```python
from build123d import *

# Parameters (mm, degrees)
SKETCH_1_W          = 20
SKETCH_1_H          = 145
EXTRUDE_1_DEPTH     = 5
SKETCH_3_W          = 20
SKETCH_3_H          = 5
EXTRUDE_2_DEPTH     = 50
SKETCH_4_W          = 20
SKETCH_4_H          = 5
EXTRUDE_3_DEPTH     = 30
SKETCH_5_W          = 20
SKETCH_5_H          = 20
CUT_EXTRUDE_1_DEPTH = 30
SKETCH_6_W          = 20
SKETCH_6_H          = 5
EXTRUDE_4_DEPTH     = 20
SKETCH_7_W          = 20
SKETCH_7_H          = 5
EXTRUDE_5_DEPTH     = 20
EXTRUDE_6_DEPTH     = 2.5
SKETCH_10_R         = 2
CUT_EXTRUDE_2_DEPTH = 5
SKETCH_11_R         = 2
CUT_EXTRUDE_3_DEPTH = 5
SKETCH_12_R         = 2.75
CUT_EXTRUDE_4_DEPTH = 5
SKETCH_13_W         = 20
SKETCH_13_H         = 5
EXTRUDE_7_DEPTH     = 5
SKETCH_14_W         = 20
SKETCH_14_H         = 5
EXTRUDE_8_DEPTH     = 20
SKETCH_15_R         = 2.75
CUT_EXTRUDE_5_DEPTH = 20
SKETCH_16_W         = 20
SKETCH_16_H         = 5
EXTRUDE_9_DEPTH     = 75.52
SKETCH_17_W         = 5
SKETCH_17_H         = 20
EXTRUDE_10_DEPTH    = 20
SKETCH_18_R         = 2.6
CUT_EXTRUDE_6_DEPTH = 20


with BuildPart() as part:
    # 草图1 → 凸台-拉伸1 (new body)
    with BuildSketch(Plane.XY):
        with Locations((0.170940171, -57.628205128)):
            Rectangle(SKETCH_1_W, SKETCH_1_H)
    extrude(amount=-EXTRUDE_1_DEPTH)

    # 草图3 → 凸台-拉伸2 (add)
    with BuildSketch(Plane(origin=(0, 0, -5), x_dir=(-1, 0, 0), z_dir=(0, 0, -1))):
        with Locations((-0.170940171, 12.371794872)):
            Rectangle(SKETCH_3_W, SKETCH_3_H)
    extrude(amount=EXTRUDE_2_DEPTH)

    # 草图4 → 凸台-拉伸3 (add)
    with BuildSketch(Plane(origin=(0, 0, -5), x_dir=(-1, 0, 0), z_dir=(0, 0, -1))):
        with Locations((-0.170940171, -107.628205128)):
            Rectangle(SKETCH_4_W, SKETCH_4_H)
    extrude(amount=EXTRUDE_3_DEPTH)

    # 草图5 → 切除-拉伸1 (cut)
    with BuildSketch(Plane(origin=(0, 0, -5), x_dir=(-1, 0, 0), z_dir=(0, 0, -1))):
        with Locations((-0.170940171, -120.128205128)):
            Rectangle(SKETCH_5_W, SKETCH_5_H)
    extrude(amount=-CUT_EXTRUDE_1_DEPTH, mode=Mode.SUBTRACT)

    # 草图6 → 凸台-拉伸4 (add)
    with BuildSketch(Plane(origin=(0, -110.128205128, 0), x_dir=(-1, 0, 0), z_dir=(0, -1, 0))):
        with Locations((-0.170940171, 32.5)):
            Rectangle(SKETCH_6_W, SKETCH_6_H)
    extrude(amount=EXTRUDE_4_DEPTH)

    # 草图7 → 凸台-拉伸5 (add)
    with BuildSketch(Plane(origin=(0, 0, -35), x_dir=(-1, 0, 0), z_dir=(0, 0, -1))):
        with Locations((-0.170940171, -127.628205128)):
            Rectangle(SKETCH_7_W, SKETCH_7_H)
    extrude(amount=EXTRUDE_5_DEPTH)

    # 草图9 → 凸台-拉伸6 (add, symmetric)
    with BuildSketch(Plane(origin=(0.170940171, 0, 0), x_dir=(0, 0, -1), z_dir=(1, 0, 0))):
        Polygon((8.965273833, -110.036991646), (29.929169638, -127.991202337), (29.929169638, -110.036991646), align=None)
    extrude(amount=EXTRUDE_6_DEPTH, both=True)

    # 草图10 → 切除-拉伸2 (cut)
    with BuildSketch(Plane.XZ.offset(-9.871794872)):
        with Locations((0.170940171, -17.5)):
            Circle(SKETCH_10_R)
        with Locations((0.170940171, -42.5)):
            Circle(SKETCH_10_R)
    extrude(amount=-CUT_EXTRUDE_2_DEPTH, mode=Mode.SUBTRACT)

    # 草图11 → 切除-拉伸3 (cut)
    with BuildSketch(Plane(origin=(0, 0, -5), x_dir=(-1, 0, 0), z_dir=(0, 0, -1))):
        with Locations((-0.170940171, -22.628205128)):
            Circle(SKETCH_11_R)
        with Locations((-0.170940171, -72.628205128)):
            Circle(SKETCH_11_R)
    extrude(amount=-CUT_EXTRUDE_3_DEPTH, mode=Mode.SUBTRACT)

    # 草图12 → 切除-拉伸4 (cut)
    with BuildSketch(Plane(origin=(0, -125.128205128, 0), x_dir=(1, 0, 0), z_dir=(0, 1, 0))):
        with Locations((0.170940171, 45)):
            Circle(SKETCH_12_R)
    extrude(amount=-CUT_EXTRUDE_4_DEPTH, mode=Mode.SUBTRACT)

    # 草图13 → 凸台-拉伸7 (add)
    with BuildSketch(Plane(origin=(0, 0, -55), x_dir=(-1, 0, 0), z_dir=(0, 0, -1))):
        with Locations((-0.170940171, -127.628205128)):
            Rectangle(SKETCH_13_W, SKETCH_13_H)
    extrude(amount=EXTRUDE_7_DEPTH)

    # 草图14 → 凸台-拉伸8 (add)
    with BuildSketch(Plane(origin=(0, -125.128205128, 0), x_dir=(1, 0, 0), z_dir=(0, 1, 0))):
        with Locations((0.170940171, 57.5)):
            Rectangle(SKETCH_14_W, SKETCH_14_H)
    extrude(amount=EXTRUDE_8_DEPTH)

    # 草图15 → 切除-拉伸5 (cut)
    with BuildSketch(Plane.XY.offset(-55)):
        with Locations((0.170940171, -115.12820513)):
            Circle(SKETCH_15_R)
    extrude(amount=-CUT_EXTRUDE_5_DEPTH, mode=Mode.SUBTRACT)

    # 草图16 → 凸台-拉伸9 (add)
    with BuildSketch(Plane(origin=(10.170940171, 0, 0), x_dir=(0, 0, -1), z_dir=(1, 0, 0))):
        with Locations((45, 12.371794872)):
            Rectangle(SKETCH_16_W, SKETCH_16_H)
    extrude(amount=EXTRUDE_9_DEPTH)

    # 草图17 → 凸台-拉伸10 (add)
    with BuildSketch(Plane(origin=(0, 14.871794872, 0), x_dir=(1, 0, 0), z_dir=(0, 1, 0))):
        with Locations((83.190940171, 45)):
            Rectangle(SKETCH_17_W, SKETCH_17_H)
    extrude(amount=EXTRUDE_10_DEPTH)

    # 草图18 → 切除-拉伸6 (cut)
    with BuildSketch(Plane.ZY.offset(-80.690940171)):
        with Locations((-45, 24.871794872)):
            Circle(SKETCH_18_R)
    extrude(amount=-CUT_EXTRUDE_6_DEPTH, mode=Mode.SUBTRACT)


solid = part.part
```
The listing builds one solid part. Answer for the finished solid, in the listing's coordinates (mm). A direction names the side the tool comes from. Give positions to 0.01 mm unless a question says otherwise; leave off trailing zeros. Order: outer loops, then holes, each group sorted by start corner. A loop starts at its lowest first (then second) coordinate and runs counter-clockwise, first axis right, second up. Notation, with made-up numbers: (-31.75, 63.5) -> (11.25, 63.5) arc R17 ccw to (11.25, 83.5) -> close; hole circle Ø10 at (41, -24.75). An arc over 180 degrees is marked (long way). Answer as a JSON object with one key per item and string values. Group by question number.
Item 1: The part is cut by section B-B on x = 6. Write down the section's boundary in (y, z), and give its area (3 significant figures).
Item 2: Flat-ended cylindrical pins translate along their axes: pin 1 (3 mm diameter, centred on x = 18, z = -39.5, fed in from +Y); pin 2 (20 mm diameter, centred on x = 33, y = 22, fed in from -Z); pin 3 (6.5 mm diameter, centred on x = 0.17, y = -22.63, fed in from -Z); pin 4 (16 mm diameter, centred on y = 21, z = -40.5, fed in from -X). Find the tip coordinate at first contact, or state that the pin passes through.
Item 3: Consider L1, parallel to Z at x = 10, y = -65.5; L2, parallel to Y at x = 82.55, z = -45; L3, parallel to Y at x = 56.5, z = -41. Determine where each line is inside the solid, lowest interval first. Write a range as from..to.
Item 4: The part is cut by section C-C on y = 20. Write down the section's boundary in (x, z).
Item 5: Determine the mould class of faces 1 (the flat face through (-9.829, -63, -3)), 2 (the cylindrical face through (-0.9, -20.94, -2.54)), 3 (the flat face through (0, -130.128, -41)), 4 (the cylindrical face through (-0.43, -117.81, -57.46)) for opening direction X: pulls with the +X half, pulls with the -X half, needs draft (parallel to the pull), parting line crosses it, or undercut.
Item 6: The part is cut by section A-A on z = -17.5. Write down the section's boundary in (x, y).
Item 7: The part is cut by section D-D on x = 29. Write down the section's boundary in (y, z), and give its area (3 significant figures).
Item 8: A tool of negligible diameter and unlimited length cuts with its end or side. For faces 5 (the flat face through (56, 14, -35)), 6 (the flat face through (3, -125.128, -43)), 7 (the flat face through (45, 14, -55)), 8 (the flat face through (25, 14.872, -39)), from which of +Z, -Z, +X, -X, +Y, -Y can it reach the whole face along a straight path? Write none if from no direction.
Result set:
{
 "1": {"outline": "(-130.13, -60) -> (-105.13, -60) -> (-105.13, -55) -> (-125.13, -55) -> (-125.13, -35) -> (-105.13, -35) -> (-105.13, -5) -> (9.87, -5) -> (9.87, -55) -> (14.87, -55) -> (14.87, 0) -> (-110.13, 0) -> (-110.13, -30) -> (-130.13, -30) -> close", "area": "1,350 mm²"},
 "2": {"pin 1": "y = 14.87", "pin 2": "z = -55", "pin 3": "z = -5", "pin 4": "x = -9.83"},
 "3": {"L1": "-5..0", "L2": "9.87..22.27, 27.47..34.87", "L3": "9.87..14.87"},
 "4": {"outline": "(80.69, -55) -> (85.69, -55) -> (85.69, -35) -> (80.69, -35) -> close"},
 "5": {"face 1": "pulls with the -X half", "face 2": "undercut", "face 3": "needs draft", "face 4": "undercut"},
 "6": {"outline": "(-9.83, -110.13) -> (-2.33, -110.13) -> (-2.33, -117.35) -> (2.67, -117.35) -> (2.67, -110.13) -> (10.17, -110.13) -> (10.17, -105.13) -> (-9.83, -105.13) -> close; (-9.83, 9.87) -> (-1.83, 9.87) -> (-1.83, 14.87) -> (-9.83, 14.87) -> close; (2.17, 9.87) -> (10.17, 9.87) -> (10.17, 14.87) -> (2.17, 14.87) -> close"},
 "7": {"outline": "(9.87, -55) -> (14.87, -55) -> (14.87, -35) -> (9.87, -35) -> close", "area": "100 mm²"},
 "8": {"face 5": "+Z, +X, +Y, -Y", "face 6": "+X, -X", "face 7": "-Z, +X, -X, +Y", "face 8": "+Z, -Z, -X, +Y"}
}
